Verification items for the finished model (mm, model axes). Face numbers are marked on the shaded views. A direction names the side the tool comes from. Give positions to 0.01 mm unless a question says otherwise; leave off trailing zeros. Loops run counter-clockwise (first coordinate to the right, second up) from the corner with the lowest first, then second, coordinate; pieces in that order, holes last. Notation, with made-up numbers: (-21, 77) - (26, 77) arc R12 ccw to (26, 92) - close; hole circle Ø10 at (-18, -6.75). An arc over 180 degrees is marked (long way). Answer in a Markdown table with one row per item.
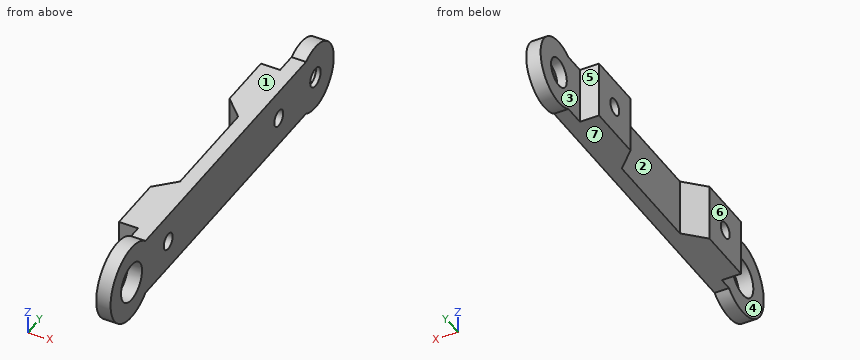
```python
from build123d import *

# Parameters (mm, degrees)
F1_DEPTH = 9.525
F2_R     = 5.55625
F2_R_2   = 6.35
F3_DEPTH = 2.38125
F4_R     = 3.175
F4_R_2   = 1.35255
F4_R_3   = 1.5875
F5_DEPTH = 5.55625
F6_R     = 2.38125
F7_DEPTH = 1.5875
F8_SIZE  = 3.17499


# Not quite as in the source:
# - a fillet or chamfer is up to 0.001 mm smaller than in the source, because OpenCascade refuses the exact size


with BuildPart() as f1:
    # F0 (on Top) → F1 (new body)
    with BuildSketch(Plane.XY):
        Polygon((0, 0), (0, 55.7060608), (-2.38125, 55.7060608), (-2.38125, 49.3560608), (-5.55625, 49.3560608), (-5.55625, 39.8310608), (-2.38125, 39.8310608), (-2.38125, 15.875), (-5.55625, 15.875), (-5.55625, 6.35), (-2.38125, 6.35), (-2.38125, 0), align=None)
    extrude(amount=F1_DEPTH)

    # F2 (on face) → F3 (join, through all)
    with BuildSketch(Plane(origin=(-2.38125, 0, 0), x_dir=(0, -1, 0), z_dir=(-1, 0, 0))):
        with Locations((-55.7060608, 4.7625)):
            Circle(F2_R)
        with Locations((0, 4.7625)):
            Circle(F2_R_2)
    extrude(amount=-F3_DEPTH)

    # F4 (on face) → F5 (cut, through all)
    with BuildSketch(Plane.YZ):
        with Locations((0, 4.7625)):
            Circle(F4_R)
        with Locations((11.1125, 4.7625)):
            Circle(F4_R_2)
        with Locations((44.5935608, 4.7625)):
            Circle(F4_R_2)
        with Locations((55.7060608001, 4.7625)):
            Circle(F4_R_3)
    extrude(amount=-F5_DEPTH, mode=Mode.SUBTRACT)

    # F6 (on face) → F7 (cut)
    with BuildSketch(Plane(origin=(-2.38125, 0, 0), x_dir=(0, -1, 0), z_dir=(-1, 0, 0))):
        with Locations((-55.7060608, 4.7625)):
            Circle(F6_R)
    extrude(amount=-F7_DEPTH, mode=Mode.SUBTRACT)

    # F8 (size 3.175 in the source; OpenCascade refuses exactly that, so slightly less here)
    f8_edges = [f1.edges().sort_by_distance(p)[0] for p in [
        (-2.38125, 39.831061, 4.7625),
        (-2.38125, 15.875, 4.7625),
    ]]
    chamfer(f8_edges, length=F8_SIZE)


solid = f1.part
```
Q1. Draft check along Y on the marked faces 5, 6 and 7. Enter one of: +Y half, -Y half, draft (parallel to the pull), parting line (faces both ways), or undercut.
Completed:
| item | result |
|---|---|
| face 5 | +Y half |
| face 6 | draft |
| face 7 | undercut |
Q2. Tool access check on the marked faces 1, 2, 3 and 4. Record the directions out of +Z, -Z, +X, -X, +Y, -Y that give a thin tool (end or side, any length) a straight path to the whole face; none if there is none.
Completed:
| item | result |
|---|---|
| face 1 | +Z, +X, -X |
| face 2 | +Z, -Z, -X |
| face 3 | +Z, -Z, -X, +Y |
| face 4 | +Z, -Z, -X, -Y |
Q3. Sectioned sample at A-A (x = -4.35). Give the number of separate pieces and of enclosed holes in the cut face, and give its area (3 significant figures).
Completed:
| item | result |
|---|---|
| separate pieces | 2 |
| enclosed holes | 2 |
| area | 193 mm^2 |
Q4. Sectioned sample at C-C (y = 45). Record the cut outline in (x, z) (3 decimals), and give its area (3 significant figures).
Completed:
| item | result |
|---|---|
| outline | (-5.556, 0) - (0, 0) - (0, 3.472) - (-5.556, 3.472) - close; (-5.556, 6.053) - (0, 6.053) - (0, 9.525) - (-5.556, 9.525) - close |
| area | 38.6 mm^2 |
Q5. Sectioned sample at B-B (y = 0). Record the cut outline in (x, z).
Completed:
| item | result |
|---|---|
| outline | (-2.38, -1.59) - (0, -1.59) - (0, 1.59) - (-2.38, 1.59) - close; (-2.38, 7.94) - (0, 7.94) - (0, 11.11) - (-2.38, 11.11) - close |
Q6. Sectioned sample at D-D (y = 22). Record the cut outline in (x, z) (3 decimals), and give its area (3 significant figures).
Completed:
| item | result |
|---|---|
| outline | (-2.381, 0) - (0, 0) - (0, 9.525) - (-2.381, 9.525) - close |
| area | 22.7 mm^2 |
Q7. Go/stop test with flat-tipped pins: P1, Ø2, axis at x = -1.5, y = 38, coming from the -Z side; P2, Ø5, axis at y = 31.5, z = 5.5, coming from the -X side; P3, Ø3, axis at x = -2.5, y = 32.5, coming from the +Z side (3 decimals). Record where each tip stops, or that it passes through.
Completed:
| item | result |
|---|---|
| P1 | z = 0 |
| P2 | x = -2.38 |
| P3 | z = 9.525 |
Q8. Thickness scan on line 1 (Y direction, x = -4.75, z = 3.75); line 2 (Z direction, x = -1.5, y = 0); line 3 (Z direction, x = -0.8, y = 30.5) (3 decimals). Record the ranges inside material, lowest first.
Completed:
| item | result |
|---|---|
| line 1 | 6.35 to 10.22, 12.01 to 16.68, 39.02 to 43.7, 45.49 to 49.36 |
| line 2 | -1.59 to 1.59, 7.94 to 11.11 |
| line 3 | 0 to 9.525 |
